from build123d import *

# Parameters (mm, degrees)
SKETCH1_R           = 1.5
BOSS_EXTRUDE1_DEPTH = 3
BOSS_EXTRUDE2_START = 12.5
SKETCH2_W           = 3.5
SKETCH2_H           = 6
BOSS_EXTRUDE2_DEPTH = 28
CHAMFER2_SIZE       = 2
SKETCH3_W           = 24
SKETCH3_H           = 28
SKETCH3_R           = 11
BOSS_EXTRUDE4_DEPTH = 6
CHAMFER3_SIZE       = 2


with BuildPart() as part:
    # Sketch1 → Boss-Extrude1 (new body)
    with BuildSketch(Plane(origin=(0, 0, 0), x_dir=(1, 0, 0), z_dir=(0, 1, 0))):
        Polygon((-6, 17), (-3, 20), (3, 20), (6, 17), (6, -17), (3, -20), (-3, -20), (-6, -17), align=None)
        with Locations(Location((0, 14, 0), (0, 0, 270))):
            Circle(SKETCH1_R, mode=Mode.SUBTRACT)
        with Locations(Location((0, -14, 0), (0, 0, 270))):
            Circle(SKETCH1_R, mode=Mode.SUBTRACT)
    extrude(amount=BOSS_EXTRUDE1_DEPTH)

    # Sketch2 → Boss-Extrude2 (add)
    with BuildSketch(Plane(origin=(0, 3, 0), x_dir=(1, 0, 0), z_dir=(0, 1, 0)).offset(BOSS_EXTRUDE2_START)):
        with Locations((-7.75, 9)):
            Rectangle(SKETCH2_W, SKETCH2_H)
        with Locations((-7.75, -9)):
            Rectangle(SKETCH2_W, SKETCH2_H)
    extrude(amount=-BOSS_EXTRUDE2_DEPTH)

    # Chamfer2
    chamfer2_edges = [part.edges().sort_by_distance(p)[0] for p in [
        (-6, 0, -9),
        (-6, 0, 9),
        (-6, 3, -9),
        (-6, 3, 9),
    ]]
    chamfer(chamfer2_edges, length=CHAMFER2_SIZE)

    # Sketch3 → Boss-Extrude4 (add)
    with BuildSketch(Plane.ZY.offset(9.5)):
        with Locations((0, 1.5)):
            Rectangle(SKETCH3_W, SKETCH3_H)
        with Locations(Location((0, 1.5, 0), (0, 0, 236.944268849))):
            Circle(SKETCH3_R, mode=Mode.SUBTRACT)
    extrude(amount=BOSS_EXTRUDE4_DEPTH)

    # Chamfer3
    chamfer3_edges = [part.edges().sort_by_distance(p)[0] for p in [
        (-10.75, 15.5, -12),
        (-10.75, -12.5, -12),
        (-10.75, -12.5, 12),
        (-10.75, 15.5, 12),
    ]]
    chamfer(chamfer3_edges, length=CHAMFER3_SIZE)


solid = part.part
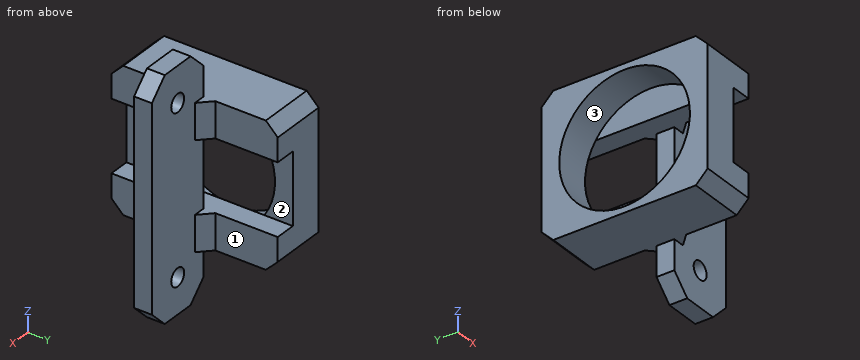
Build history of the part. All positions in model axes, mm. Face numbers are marked on the shaded views. A direction names the side the tool comes from. Coordinates: 2 decimals unless noted, no trailing zeros. Write each loop counter-clockwise with the first axis right and the second up, starting at its lowest first coordinate (ties: lowest second). Pieces come first, ordered by that corner, then holes. Notation, with made-up numbers: (-18, 33) -> (-8, 33) arc R35 ccw to (-8, 68) -> close; hole circle Ø11 at (76.25, 53). An arc over 180 degrees is marked (long way). Use CSV: the item, a comma, the result in double quotes. Start each with the question number.
Q1. Drill centre lines: probe 1 along Z at (x, y) = (-6.75, 4); probe 2 along Z at (x, y) = (-13.3, 1.5); probe 3 along Y at (x, z) = (-12.7, 0). Where is each one in solid material? Low to high.
Q2. Cut at D-D, the plane x = 0. List the corners of the cut face in (y, z), then the cut area to 3 significant figures.
Q3. Cut at A-A, the plane x = -7.5. List the corners of the cut face in (y, z), then the cut area to 3 significant figures.
Q4. Cut at C-C, the plane z = 14. List the corners of the cut face in (x, y).
Q5. Cut at B-B, the plane y = 1.5. List the corners of the cut face in (x, z), then the cut area to 3 significant figures.
Q6. Flat gauge pins, fed straight in: pin 1 Ø5 at (x, y) = (-12, 2) entering from +Z; pin 2 Ø5 at (y, z) = (9.5, 8) entering from +X; pin 3 Ø6 at (x, z) = (-2.5, -2) entering from +Y; pin 4 Ø2.5 at (x, z) = (0, -14) entering from +Y. Where does each tip first touch, or does it go through?
Q7. 3-axis set-ups, long thin cutter, end or side, ignore diameter. For the marked faces 1, 2 and 3: which of +Z, -Z, +X, -X, +Y, -Y reach the whole face in a straight line?
Checked values:
1,probe 1,"z = -12 to -6, 6 to 12"
1,probe 2,"z = -12 to -11, 11 to 12"
1,probe 3,"y = -12.5 to -9.5, 12.5 to 15.5"
2,outline,"(0, -20) -> (3, -20) -> (3, -15.5) -> (0, -15.5) -> close; (0, -12.5) -> (3, -12.5) -> (3, 12.5) -> (0, 12.5) -> close; (0, 15.5) -> (3, 15.5) -> (3, 20) -> (0, 20) -> close"
2,area,"102 mm²"
3,outline,"(-12.5, -10) -> (-10.5, -12) -> (13.5, -12) -> (15.5, -10) -> (15.5, -6) -> (-12.5, -6) -> close; (-12.5, 6) -> (15.5, 6) -> (15.5, 10) -> (13.5, 12) -> (-10.5, 12) -> (-12.5, 10) -> close"
3,area,"328 mm²"
4,outline,"(-6, 0) -> (-1.5, 0) -> (-1.5, 3) -> (-6, 3) -> close; (1.5, 0) -> (6, 0) -> (6, 3) -> (1.5, 3) -> close"
5,outline,"(-15.5, -12) -> (-6, -12) -> (-6, -17) -> (-3, -20) -> (3, -20) -> (6, -17) -> (6, 17) -> (3, 20) -> (-3, 20) -> (-6, 17) -> (-6, 12) -> (-15.5, 12) -> (-15.5, 11) -> (-9.5, 11) -> (-9.5, 6) -> (-6, 6) -> (-6, -6) -> (-9.5, -6) -> (-9.5, -11) -> (-15.5, -11) -> close; hole circle Ø3 at (0, -14); hole circle Ø3 at (0, 14)"
5,area,"502 mm²"
6,pin 1,"stops at z = 12"
6,pin 2,"stops at x = -6"
6,pin 3,"stops at y = 3"
6,pin 4,"passes through"
7,face 1,"+Z, -Z, +X, +Y"
7,face 2,"+X, +Y, -Y"
7,face 3,"-X"
